Check sheet for the modelled part. Datum: model origin and axes. Units: mm. A direction names the side the tool comes from. Coordinates: 2 decimals unless noted, no trailing zeros. Loops run counter-clockwise (first coordinate to the right, second up) from the corner with the lowest first, then second, coordinate; pieces in that order, holes last.
```python
from build123d import *

# Parameters (mm, degrees)
SKETCH_R        = 2.25
SKETCH_R_2      = 11.25
SKETCH_R_3      = 1.75
PAD_DEPTH       = 20.7
POCKET_DEPTH    = 17.7
SKETCH002_R     = 4
PAD001_DEPTH    = 8
SKETCH003_R     = 3
POCKET001_DEPTH = 8
SKETCH004_R     = 1.75
POCKET002_DEPTH = 5
SKETCH005_R     = 4.05
POCKET003_DEPTH = 12
SKETCH006_R     = 1.75
POCKET004_DEPTH = 12.701


with BuildPart() as pocket_belt_path:
    # Sketch → Pad (new body)
    with BuildSketch(Plane.XY):
        Polygon((0, 0), (105, 0), (105, 62), (20, 62), (20, 42), (0, 42), align=None)
        with Locations((38, 10)):
            Circle(SKETCH_R, mode=Mode.SUBTRACT)
        with Locations((33, 35)):
            Circle(SKETCH_R, mode=Mode.SUBTRACT)
        with Locations((84, 21)):
            Circle(SKETCH_R_2, mode=Mode.SUBTRACT)
        with Locations((68.5, 36.5)):
            Circle(SKETCH_R_3, mode=Mode.SUBTRACT)
        with Locations((99.5, 36.5)):
            Circle(SKETCH_R_3, mode=Mode.SUBTRACT)
        with Locations((68.5, 5.5)):
            Circle(SKETCH_R_3, mode=Mode.SUBTRACT)
        with Locations((99.5, 5.5)):
            Circle(SKETCH_R_3, mode=Mode.SUBTRACT)
        with Locations((10, 30)):
            Circle(SKETCH_R, mode=Mode.SUBTRACT)
        with Locations((10, 15)):
            Circle(SKETCH_R, mode=Mode.SUBTRACT)
        with Locations((42, 52)):
            Circle(SKETCH_R, mode=Mode.SUBTRACT)
        with Locations((94, 52)):
            Circle(SKETCH_R, mode=Mode.SUBTRACT)
        with Locations((55, 5)):
            Circle(SKETCH_R_3, mode=Mode.SUBTRACT)
        with BuildLine():
            Line((58.75, 25.000001), (58.75, 40))
            ThreePointArc((58.75, 40), (56.5, 42.25), (54.25, 39.999999))
            Line((54.25, 25), (54.25, 39.999999))
            ThreePointArc((54.25, 25), (56.5, 22.75), (58.75, 25.000001))
        make_face(mode=Mode.SUBTRACT)
    extrude(amount=PAD_DEPTH)

    # Sketch001 → Pocket (cut)
    with BuildSketch(Plane.XY.offset(20.7)):
        with BuildLine():
            ThreePointArc((41.485277, 42), (39.015593, 44.209375), (35.999996, 45.583005))
            Line((35.999996, 67), (35.999996, 45.583005))
            Line((20, 67), (35.999996, 67))
            Line((20, -1), (20, 67))
            Line((20, -1), (48.252269, -1))
            Line((48.252269, 11), (48.252269, -1))
            Line((48.252269, 11), (70.252269, 11))
            ThreePointArc((70.252269, 11), (71.759618, 9.202833), (73.499996, 7.630258))
            Line((73.499996, 7.630258), (73.499996, -1))
            Line((73.499996, -1), (93.499996, -1))
            Line((93.499996, -1), (93.499996, 6.902128))
            ThreePointArc((93.499996, 6.902128), (95.574295, 8.548671), (97.367695, 10.497399))
            Line((105.499996, 10.497399), (97.367695, 10.497399))
            Line((105.499996, 30.497399), (105.499996, 10.497399))
            Line((98.099621, 30.497399), (105.499996, 30.497399))
            ThreePointArc((98.099621, 30.497399), (91.98574, 36.007594), (83.999996, 38))
            Line((83.999996, 38), (83.999996, 67))
            Line((83.999996, 67), (46.999996, 67))
            Line((46.999996, 67), (46.999996, 42))
            Line((41.485277, 42), (46.999996, 42))
        make_face()
    extrude(amount=-POCKET_DEPTH, mode=Mode.SUBTRACT)


with BuildPart() as pocket004:
    # Part__Mirroring: instance of Pocket belt path
    add(pocket_belt_path.part.mirror(Plane(origin=(52.5, 31, 0), x_dir=(0, 1, 0), z_dir=(0, 0, 1))))

    # Sketch002 → Pad001 (new body)
    with BuildSketch(Plane(origin=(0, 0, -3), x_dir=(1, 0, 0), z_dir=(0, 0, -1))):
        with Locations((68.5, -36.5)):
            Circle(SKETCH002_R)
    extrude(amount=PAD001_DEPTH)

    # Sketch003 → Pocket001 (cut)
    with BuildSketch(Plane.XY):
        with Locations((55, 5)):
            Circle(SKETCH003_R)
        with Locations((68.5, 36.5)):
            Circle(SKETCH003_R)
        with Locations((68.5, 5.5)):
            Circle(SKETCH003_R)
        with Locations((99.5, 36.5)):
            Circle(SKETCH003_R)
        with Locations((99.5, 5.5)):
            Circle(SKETCH003_R)
    extrude(amount=-POCKET001_DEPTH, mode=Mode.SUBTRACT)

    # Sketch004 → Pocket002 (cut)
    with BuildSketch(Plane.XY.offset(-8)):
        with Locations((94, 52)):
            Circle(SKETCH004_R)
    extrude(amount=-POCKET002_DEPTH, mode=Mode.SUBTRACT)

    # Sketch005 → Pocket003 (cut)
    with BuildSketch(Plane.XZ):
        with Locations((13, -20.7)):
            Circle(SKETCH005_R)
    extrude(amount=-POCKET003_DEPTH, mode=Mode.SUBTRACT)

    # Sketch006 → Pocket004 (cut, through all)
    with BuildSketch(Plane.XY.offset(-8)):
        with Locations((68.5, 36.5)):
            Circle(SKETCH006_R)
    extrude(amount=-POCKET004_DEPTH, mode=Mode.SUBTRACT)


solid = pocket004.part
```
1) Section check C-C on x = 68.5. Enter the section's corners in (y, z).
Answer sheet:
outline: (0, -20.7) - (3.75, -20.7) - (3.75, -8) - (2.5, -8) - (2.5, 0) - (0, 0) - close; (7.25, -20.7) - (11, -20.7) - (11, -3) - (32.5, -3) - (32.5, -11) - (34.75, -11) - (34.75, -8) - (33.5, -8) - (33.5, 0) - (8.5, 0) - (8.5, -8) - (7.25, -8) - close; (38.25, -11) - (40.5, -11) - (40.5, -3) - (62, -3) - (62, 0) - (39.5, 0) - (39.5, -8) - (38.25, -8) - close
2) Set-up check for faces 1 (the flat face through (93.5, 3, -12)), 2 (the flat face through (69.33, 38.22, -11)), 3 (the cylindrical face through (56.55, 42.25, -1.48)), 4 (the flat face through (101, 4, -8)): record each of +Z, -Z, +X, -X, +Y, -Y from which the full face is reachable in a straight line by a thin tool's end or side.
Answer sheet:
face 1: -Z, -Y
face 2: -Z, +Y
face 3: +Z, -Z
face 4: +Z
3) Section check D-D on y = 26.5. Enter the section's corners in (x, z).
Answer sheet:
outline: (0, -20.7) - (20, -20.7) - (20, -3) - (54.25, -3) - (54.25, 0) - (0, 0) - close; (58.75, -3) - (74.19, -3) - (74.19, 0) - (58.75, 0) - close; (93.81, -3) - (105, -3) - (105, 0) - (93.81, 0) - close
4) Section check B-B on x = 33. Enter the section's corners in (y, z), plus the area to 4 significant figures.
Answer sheet:
outline: (0, -3) - (32.75, -3) - (32.75, 0) - (0, 0) - close; (37.25, -3) - (62, -3) - (62, 0) - (37.25, 0) - close
area: 172.5 mm2
5) Mould release check, pull along X, two halves, no side actions. Record for faces 5 (the cylindrical face through (39.21, 11.897, -1.479)), 6 (the flat face through (10, 26, -20.7)): +X half, -X half, draft (parallel to the pull), parting line (faces both ways), or undercut.
Answer sheet:
face 5: undercut
face 6: draft
6) Section check A-A on z = -13.5. Give the number of separate pieces and of enclosed holes in the cut face, plus the area to 3 significant figures.
Answer sheet:
separate pieces: 5
enclosed holes: 8
area: 1,920 mm2
7) Scan lines: line 1 (Y direction, x = 99.5, z = -10.75); line 2 (Y direction, x = 33, z = -1.7); line 3 (X direction, y = 48.5, z = -6.5). Record each from-to range of solid material in increasing order.
Answer sheet:
line 1: y = 0 to 3.75, 7.25 to 10.5, 30.5 to 34.75, 38.25 to 62
line 2: y = 0 to 32.75, 37.25 to 62
line 3: x = 36 to 47, 84 to 105
8) Depth check by flat-ended pin: pin 1 (0.9 mm diameter, centred on y = 56, z = -1.5, fed in from -X); pin 2 (2.5 mm diameter, centred on x = 67, y = 37.5, fed in from -Z); pin 3 (6 mm diameter, centred on x = 70.5, z = -11.5, fed in from +Y). Enter the tip coordinate at first touch or a pass-through.
Answer sheet:
pin 1: stops at x = 20
pin 2: stops at z = -11
pin 3: stops at y = 40.5
